from build123d import *

# Parameters (mm, degrees)
SKETCH1_W               = 50
SKETCH1_H               = 50
BOSS_EXTRUDE1_DEPTH     = 6
SKETCH2_R               = 15
BOSS_EXTRUDE2_DEPTH     = 36.7
CHAMFER1_SIZE           = 7
CUT_EXTRUDE1_DEPTH      = 36.7
CUT_EXTRUDE1_DEPTH_BACK = 36.7
SKETCH3_W               = 10
SKETCH3_H               = 35.728035611
CUT_EXTRUDE2_DEPTH      = 36.7
CUT_EXTRUDE2_DEPTH_BACK = 36.7
CUT_EXTRUDE3_DEPTH      = 36.7
CUT_EXTRUDE3_DEPTH_BACK = 36.7
SKETCH5_R               = 5
SKETCH7_R               = 1.5
CUT_EXTRUDE4_DEPTH      = 9
CHAMFER2_SIZE           = 7


with BuildPart() as part:
    # Sketch1 → Boss-Extrude1 (new body)
    with BuildSketch(Plane(origin=(0, 0, 0), x_dir=(1, 0, 0), z_dir=(0, 1, 0))):
        Rectangle(SKETCH1_W, SKETCH1_H)
    extrude(amount=BOSS_EXTRUDE1_DEPTH)

    # Sketch2 → Boss-Extrude2 (add)
    with BuildSketch(Plane(origin=(0, 6, 0), x_dir=(1, 0, 0), z_dir=(0, 1, 0))):
        with Locations(Location((0, 0, 0), (0, 0, 270))):
            Circle(SKETCH2_R)
    extrude(amount=BOSS_EXTRUDE2_DEPTH)

    # Chamfer1
    chamfer1_edges = [part.edges().sort_by_distance(p)[0] for p in [
        (25, 3, 25),
    ]]
    chamfer(chamfer1_edges, length=CHAMFER1_SIZE)

    # Sketch3 → Cut-Extrude1 (cut, two sides: drawn at the far end of the back side and taken through both)
    with BuildSketch(Plane.XY.offset(-CUT_EXTRUDE1_DEPTH_BACK)):
        with Locations((0, 25.764017805)):
            Rectangle(SKETCH3_W, SKETCH3_H)
    extrude(amount=CUT_EXTRUDE1_DEPTH + CUT_EXTRUDE1_DEPTH_BACK, mode=Mode.SUBTRACT)

    # Sketch4 → Cut-Extrude2 (cut, two sides: drawn at the far end of the back side and taken through both)
    with BuildSketch(Plane(origin=(0, 0, 0), x_dir=(0, 0, -1), z_dir=(1, 0, 0)).offset(-CUT_EXTRUDE2_DEPTH_BACK)):
        with BuildLine():
            Line((-14.375997607, 31.981435834), (-17.281195567, 49.289848302))
            Line((-17.281195567, 49.289848302), (26.224300548, 49.289848302))
            Line((26.224300548, 49.289848302), (14.47548732, 31.631954585))
            ThreePointArc((14.47548732, 31.631954585), (0.181683341, 42.698899665), (-14.375997607, 31.981435834))
        make_face()
    extrude(amount=CUT_EXTRUDE2_DEPTH + CUT_EXTRUDE2_DEPTH_BACK, mode=Mode.SUBTRACT)

    # Sketch5 → Cut-Extrude3 (cut, two sides: drawn at the far end of the back side and taken through both)
    with BuildSketch(Plane(origin=(0, 0, 0), x_dir=(0, 0, -1), z_dir=(1, 0, 0)).offset(-CUT_EXTRUDE3_DEPTH_BACK)):
        with Locations(Location((0, 26, 0), (0, 0, 180))):
            Circle(SKETCH5_R)
    extrude(amount=CUT_EXTRUDE3_DEPTH + CUT_EXTRUDE3_DEPTH_BACK, mode=Mode.SUBTRACT)

    # Sketch6 → Revolve1 (revolve)
    with BuildSketch(Plane(origin=(0, 0, 0), x_dir=(0, 0, -1), z_dir=(1, 0, 0))):
        with BuildLine():
            Line((-15, 7.9), (-15, 6))
            Line((-15, 6), (-16.9, 6))
            ThreePointArc((-16.9, 6), (-16.343502884, 7.343502884), (-15, 7.9))
        make_face()
    revolve(axis=Axis((0, 42.7, 0), (0, -1, 0)))

    # Sketch7 → Cut-Extrude4 (cut)
    with BuildSketch(Plane(origin=(0, 6, 0), x_dir=(1, 0, 0), z_dir=(0, 1, 0))):
        with Locations(Location((-18.5, 18.5, 0), (0, 0, 270))):
            Circle(SKETCH7_R)
        with Locations(Location((18.5, 18.5, 0), (0, 0, 270))):
            Circle(SKETCH7_R)
        with Locations(Location((18.5, -18.5, 0), (0, 0, 270))):
            Circle(SKETCH7_R)
        with Locations(Location((-18.5, -18.5, 0), (0, 0, 270))):
            Circle(SKETCH7_R)
    extrude(amount=-CUT_EXTRUDE4_DEPTH, mode=Mode.SUBTRACT)

    # Chamfer2
    chamfer2_edges = [part.edges().sort_by_distance(p)[0] for p in [
        (-25, 3, 25),
    ]]
    chamfer(chamfer2_edges, length=CHAMFER2_SIZE)


solid = part.part
Design review of the part built by this model. Coordinates are the model's own, in mm. A direction names the side the tool comes from. Give positions to 0.01 mm unless a question says otherwise; leave off trailing zeros. Write each loop counter-clockwise with the first axis right and the second up, starting at its lowest first coordinate (ties: lowest second). Pieces come first, ordered by that corner, then holes. Notation, with made-up numbers: M -37.5,64 L -14.5,64 A32 cw -14.5,97 Z; hole C 8,-28.75 d4. An arc over 180 degrees is marked long. Return JSON: item names as keys, results as strings. Group by question number.
Item 1: Tool access review of faces 4 (the flat face through (-6, 6, -17)), 5 (the cylindrical face through (-14.51, 21.19, 3.8)), 6 (the cylindrical face through (-18.43, 3.04, 17)), 7 (the flat face through (0, 7.9, 0)), 8 (the flat face through (-22, 3, 21)): name each direction out of +Z, -Z, +X, -X, +Y, -Y from which nothing blocks a thin tool from reaching the whole face with its end or side.
Item 2: Take a section at A-A (z = -18.5). Give the boundary of the cut face in (x, y), plus the area to 3 significant figures.
Item 3: Wall thickness on line 1 along X through (y, z) = (1.2, -18.5); line 2 along X through (y, z) = (1, -18); line 3 along Y through (x, z) = (-11, 0): over which ranges is each line inside the solid? List them lowest first.
Item 4: Take a section at C-C (y = 37). Give the boundary of the cut face in (x, z), plus the area to 3 significant figures.
Item 5: The part is to be moulded in two halves that separate along X. For faces 1 (the cylindrical face through (14.51, 21.19, -3.8)), 2 (the cylindrical face through (-10.073, 21.043, -0.651)), 3 (the flat face through (-5, 21, 3)), say which applies: pulls with the +X half, pulls with the -X half, needs draft (parallel to the pull), parting line crosses it, or undercut.
Item 6: Take a section at D-D (y = 12.5). Give the boundary of the cut face in (x, z).
Item 7: Take a section at B-B (y = 26). Give the boundary of the cut face in (x, z), plus the area to 3 significant figures.
Item 8: Clearance check with flat-ended pins moving along their axes: pin 1 Ø4 at (x, y) = (2.5, 37) entering from -Z; pin 2 Ø8 at (x, y) = (5.5, 37.5) entering from -Z; pin 3 Ø2 at (x, z) = (13.5, -15.5) entering from +Y; pin 4 Ø14 at (y, z) = (18.5, -6.5) entering from +X. State where each tip first meets the part, or that it passes through.
Return value:
{
 "1": {"face 4": "+Y", "face 5": "-X, +Y", "face 6": "+Y, -Y", "face 7": "+Z, -Z, +Y", "face 8": "+Z, -X, +Y, -Y"},
 "2": {"outline": "M -25,0 L -20,0 L -20,6 L -25,6 Z; M -17,0 L 17,0 L 17,6 L -17,6 Z; M 20,0 L 25,0 L 25,6 L 20,6 Z", "area": "264 mm2"},
 "3": {"line 1": "x = -25 to -20, -17 to 17, 20 to 25", "line 2": "x = -25 to -19.91, -17.09 to 17.09, 19.91 to 25", "line 3": "y = 0 to 21, 31 to 42.7"},
 "4": {"outline": "M -9.3,-11.77 L -5,-11.77 L -5,11.77 L -9.3,11.77 A15 ccw Z; M 5,-11.77 L 9.3,-11.77 A15 ccw 9.3,11.77 L 5,11.77 Z", "area": "389 mm2"},
 "5": {"face 1": "pulls with the +X half", "face 2": "needs draft", "face 3": "undercut"},
 "6": {"outline": "M -5,-14.14 L -5,14.14 A15 ccw Z; M 5,-14.14 A15 ccw 5,14.14 Z"},
 "7": {"outline": "M -14.14,-5 A15 ccw -5,-14.14 L -5,-5 Z; M -14.14,5 L -5,5 L -5,14.14 A15 ccw Z; M 5,-14.14 A15 ccw 14.14,-5 L 5,-5 Z; M 5,5 L 14.14,5 A15 ccw 5,14.14 Z", "area": "218 mm2"},
 "8": {"pin 1": "passes through", "pin 2": "stops at z = -13.83", "pin 3": "stops at y = 6", "pin 4": "stops at x = 15"}
}
